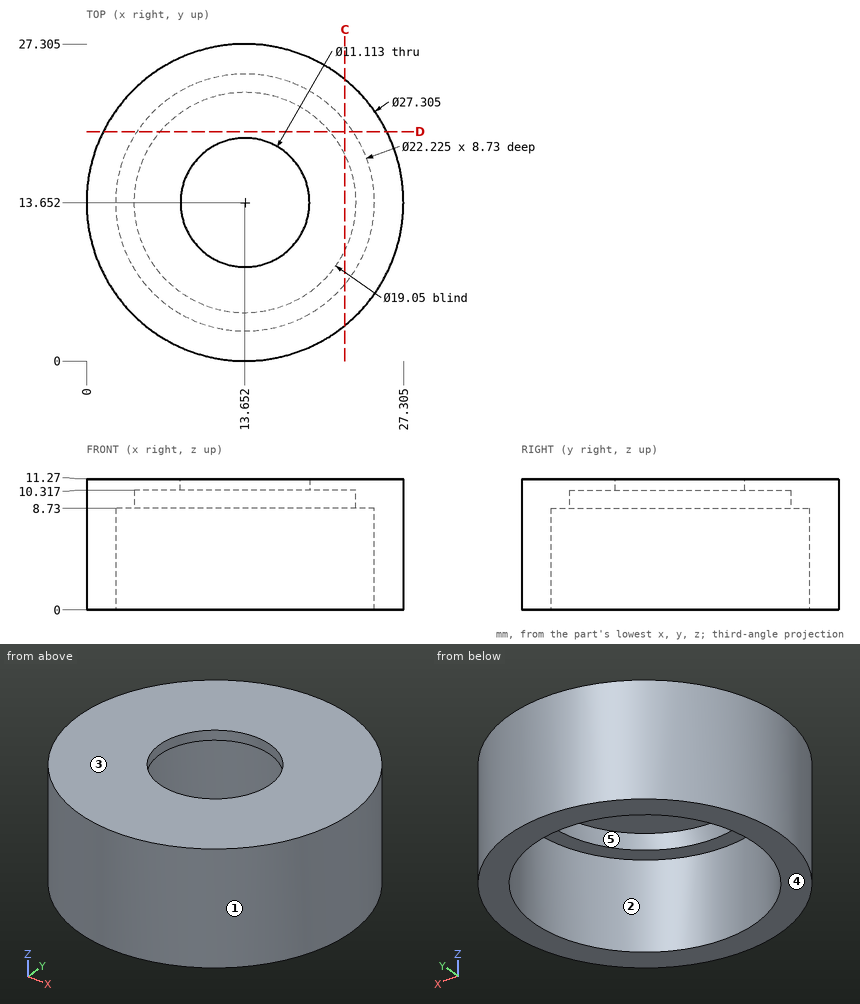
Geometry check sheet. Reference: drawing and pictorial views, mm from the part's lowest x, y, z. A direction names the side the tool comes from. Coordinates: 2 decimals unless noted, no trailing zeros. Order: outer loops, then holes, each group sorted by start corner. A loop starts at its lowest first (then second) coordinate and runs counter-clockwise, first axis right, second up. Notation, with made-up numbers: (33, -9.5) - (58, -9.5) arc R10 ccw to (58, -3.5) - close; hole circle Ø8 at (-39, 48.25). An arc over 180 degrees is marked (long way). Answer in a Markdown table with one row per item. Add a question column.
1) Release check for a two-part mould opening along X. For the marked faces 1, 2 and 3 record: +X half, -X half, draft (parallel to the pull), parting line (faces both ways), or undercut.
2) Cross-section at C-C, the plane x = 22.25. Record the cut outline in (y, z), then the cut area to 3 significant figures.
3) Cross-section at D-D, the plane y = 19.75. Record the cut outline in (x, z) (1 decimal).
4) Gauge pin test, flat ends, axial feed: P1, Ø5, axis at x = 8.5, z = 5.5, coming from the -Y side; P2, Ø6.5, axis at x = 11.5, y = 16, coming from the -Z side; P3, Ø4, axis at y = 3, z = 8, coming from the -X side. Record the tip position at first contact, or that the pin passes through.
5) Set-up check for the marked faces 4 and 5: record each of +Z, -Z, +X, -X, +Y, -Y from which the full face is reachable in a straight line by a thin tool's end or side.
6) Material ranges on line 1 along X through (y, z) = (13.75, 5.75) (1 decimal); line 2 along Y through (x, z) = (11, 9.25) (1 decimal), recorded low to high. Write a range as [from, to].
Check result:
| question | item | result |
|---|---|---|
| 1 | face 1 | parting line |
| 1 | face 2 | undercut |
| 1 | face 3 | draft |
| 2 | outline | (3.05, 0) - (6.61, 0) - (6.61, 8.73) - (9.55, 8.73) - (9.55, 10.32) - (17.75, 10.32) - (17.75, 8.73) - (20.69, 8.73) - (20.69, 0) - (24.26, 0) - (24.26, 11.27) - (3.05, 11.27) - close |
| 2 | area | 103 mm² |
| 3 | outline | (1.4, 0) - (4.4, 0) - (4.4, 8.7) - (6.3, 8.7) - (6.3, 10.3) - (21, 10.3) - (21, 8.7) - (22.9, 8.7) - (22.9, 0) - (25.9, 0) - (25.9, 11.3) - (1.4, 11.3) - close |
| 4 | P1 | stops at y = 0.26 |
| 4 | P2 | stops at z = 10.32 |
| 4 | P3 | stops at x = 3.09 |
| 5 | face 4 | -Z, +X, -X, +Y, -Y |
| 5 | face 5 | -Z |
| 6 | line 1 | x = [0, 2.5], [24.8, 27.3] |
| 6 | line 2 | y = [0.3, 4.5], [22.8, 27] |
